Geometry: final body of the model. Coordinates: model frame, mm. A direction names the side the tool comes from. Coordinates: 2 decimals unless noted, no trailing zeros. Loops run counter-clockwise (first coordinate to the right, second up) from the corner with the lowest first, then second, coordinate; pieces in that order, holes last. Notation, with made-up numbers: (56, -6) - (65, -6) arc R27 cw to (65, 16) - close; hole circle Ø7 at (-40, 12.5). An arc over 180 degrees is marked (long way). Answer in a Markdown table with one row per item.
from build123d import *

# Parameters (mm, degrees)
BOSS_EXTRUDE1_DEPTH     = 19.05
SKETCH2_W               = 42.164
SKETCH2_H               = 27.686
BOSS_EXTRUDE2_DEPTH     = 2.54
SKETCH3_W               = 7.0612
SKETCH3_H               = 14.986
BOSS_EXTRUDE3_DEPTH     = 3.175
CUT_EXTRUDE1_DEPTH      = 50.127067096
CUT_EXTRUDE1_DEPTH_BACK = 50.127067096
SKETCH4_R               = 1.75
FILLET2_R               = 1.27
CUT_EXTRUDE2_DEPTH      = 52.65763053
CUT_EXTRUDE2_DEPTH_BACK = 52.65763053
SKETCH5_R               = 4.7625
SKETCH6_W               = 25.4
SKETCH6_H               = 4.7625
BOSS_EXTRUDE4_DEPTH     = 9.525
FILLET3_R               = 3.175
FILLET4_R               = 1.27
FILLET6_R               = 1.27
SKETCH8_R               = 2.3
CUT_EXTRUDE3_DEPTH      = 58.486687197
SKETCH9_W               = 2.54
SKETCH9_H               = 10.16
CUT_EXTRUDE4_DEPTH      = 14.5288
FILLET3_OF_MIRROR2_R    = 3.175
FILLET4_OF_MIRROR2_R    = 1.27
SKETCH11_W              = 43.835439061
SKETCH11_H              = 10.898597795
CUT_EXTRUDE5_DEPTH      = 6.858


with BuildPart() as part:
    # Sketch1 → Boss-Extrude1 (new body)
    with BuildSketch(Plane.XY):
        Polygon((-2.54, 25.146), (39.624, 25.146), (39.624, 22.606), (37.084, 22.606), (0, 22.606), (0, 0), (37.084, 0), (39.624, 0), (39.624, -2.54), (-2.54, -2.54), align=None)
    extrude(amount=BOSS_EXTRUDE1_DEPTH)

    # Sketch2 → Boss-Extrude2 (add)
    with BuildSketch(Plane.XY.offset(19.05)):
        with Locations((18.542, 11.303)):
            Rectangle(SKETCH2_W, SKETCH2_H)
    extrude(amount=BOSS_EXTRUDE2_DEPTH)

    # Sketch3 → Boss-Extrude3 (add)
    with BuildSketch(Plane.ZY.offset(2.54)):
        with Locations((18.0594, 11.303)):
            Rectangle(SKETCH3_W, SKETCH3_H)
    extrude(amount=BOSS_EXTRUDE3_DEPTH)

    # Sketch4 → Cut-Extrude1 (cut, two sides: drawn at the far end of the back side and taken through both)
    with BuildSketch(Plane(origin=(0, 0, 14.5288), x_dir=(-1, 0, 0), z_dir=(0, 0, -1)).offset(-CUT_EXTRUDE1_DEPTH_BACK)):
        with Locations(Location((2.2225, 11.303, 0), (0, 0, 90))):
            Circle(SKETCH4_R)
    extrude(amount=CUT_EXTRUDE1_DEPTH + CUT_EXTRUDE1_DEPTH_BACK, mode=Mode.SUBTRACT)

    # Fillet2
    fillet2_edges = [part.edges().sort_by_distance(p)[0] for p in [
        (-2.54, 18.796, 18.0594),
        (-2.54, 3.81, 18.0594),
        (-5.715, 18.796, 18.0594),
        (-5.715, 3.81, 18.0594),
    ]]
    fillet(fillet2_edges, radius=FILLET2_R)

    # Sketch5 → Cut-Extrude2 (cut, two sides: drawn at the far end of the back side and taken through both)
    with BuildSketch(Plane.XY.offset(21.59).offset(-CUT_EXTRUDE2_DEPTH_BACK)):
        with Locations((10.16, 11.303)):
            Circle(SKETCH5_R)
        with BuildLine():
            Line((25.4, 16.0655), (10.16, 16.0655))
            ThreePointArc((10.16, 16.0655), (13.527596045, 14.670596045), (14.9225, 11.303))
            ThreePointArc((14.9225, 11.303), (13.527596045, 7.935403955), (10.16, 6.5405))
            Line((10.16, 6.5405), (25.4, 6.5405))
            ThreePointArc((25.4, 6.5405), (20.6375, 11.303), (25.4, 16.0655))
        make_face()
        with Locations((25.4, 11.303)):
            Circle(SKETCH5_R)
    extrude(amount=CUT_EXTRUDE2_DEPTH + CUT_EXTRUDE2_DEPTH_BACK, mode=Mode.SUBTRACT)

    # Sketch6 → Boss-Extrude4 (add)
    with BuildSketch(Plane.XY.offset(21.59)):
        with Locations((26.924, 22.76475)):
            Rectangle(SKETCH6_W, SKETCH6_H)
    boss_extrude4 = extrude(amount=BOSS_EXTRUDE4_DEPTH)

    # Fillet3
    fillet3_edges = [part.edges().sort_by_distance(p)[0] for p in [
        (14.224, 22.76475, 21.59),
        (14.224, 22.76475, 31.115),
        (39.624, 22.76475, 31.115),
    ]]
    fillet(fillet3_edges, radius=FILLET3_R)

    # Fillet4
    fillet4_edges = [part.edges().sort_by_distance(p)[0] for p in [
        (25.3365, 20.3835, 21.59),
    ]]
    fillet(fillet4_edges, radius=FILLET4_R)

    # Fillet6
    fillet6_edges = [part.edges().sort_by_distance(p)[0] for p in [
        (0, 0, 9.525),
        (0, 22.606, 9.525),
    ]]
    fillet(fillet6_edges, radius=FILLET6_R)

    # Sketch8 → Cut-Extrude3 (cut, symmetric)
    with BuildSketch(Plane(origin=(0, 25.146, 0), x_dir=(1, 0, 0), z_dir=(0, 1, 0))):
        with Locations(Location((20.574, -26.3525, 0), (0, 0, 270))):
            Circle(SKETCH8_R)
        with Locations(Location((33.274, -26.3525, 0), (0, 0, 270))):
            Circle(SKETCH8_R)
    cut_extrude3 = extrude(amount=CUT_EXTRUDE3_DEPTH, both=True, mode=Mode.SUBTRACT)

    # Sketch9 → Cut-Extrude4 (cut)
    with BuildSketch(Plane(origin=(0, 0, 0), x_dir=(-1, 0, 0), z_dir=(0, 0, -1))):
        with Locations((1.27, 11.303)):
            Rectangle(SKETCH9_W, SKETCH9_H)
    extrude(amount=-CUT_EXTRUDE4_DEPTH, mode=Mode.SUBTRACT)

    # Mirror2: Boss-Extrude4, Cut-Extrude3 across plane
    add(boss_extrude4.mirror(Plane.ZX.offset(11.303)))
    add(cut_extrude3.mirror(Plane.ZX.offset(11.303)), mode=Mode.SUBTRACT)

    # Fillet3 of Mirror2
    fillet3_of_mirror2_edges = [part.edges().sort_by_distance(p)[0] for p in [
        (14.224, -0.15875, 21.59),
        (14.224, -0.15875, 31.115),
        (39.624, -0.15875, 31.115),
    ]]
    fillet(fillet3_of_mirror2_edges, radius=FILLET3_OF_MIRROR2_R)

    # Fillet4 of Mirror2
    fillet4_of_mirror2_edges = [part.edges().sort_by_distance(p)[0] for p in [
        (25.3365, 2.2225, 21.59),
    ]]
    fillet(fillet4_of_mirror2_edges, radius=FILLET4_OF_MIRROR2_R)

    # Sketch11 → Cut-Extrude5 (cut)
    with BuildSketch(Plane(origin=(0, 25.146, 0), x_dir=(1, 0, 0), z_dir=(0, 1, 0))):
        with Locations((19.377719531, -27.039298898)):
            Rectangle(SKETCH11_W, SKETCH11_H)
    extrude(amount=-CUT_EXTRUDE5_DEPTH, mode=Mode.SUBTRACT)


solid = part.part
(1) Pull-direction query (Y, two-part tool) for faces 6 (the face through (-3.93, 10.92, 18.11)), 7 (the face through (38.67, -0.19, 30.21)), 8 (the face through (-5.33, 4.17, 18.11)), 9 (the face through (21, 0, 9)); classes: pulls with the +Y half, pulls with the -Y half, needs draft (parallel to the pull), parting line crosses it, or undercut.
Verdict:
| item | result |
|---|---|
| face 6 | undercut |
| face 7 | needs draft |
| face 8 | pulls with the -Y half |
| face 9 | undercut |
(2) Ray query, probe 1 along Y at (x, z) = (37, 10.5); probe 2 along Y at (x, z) = (-1, 3); probe 3 along X at (y, z) = (20.5, 4). Return the intervals inside material, ascending.
Verdict:
| item | result |
|---|---|
| probe 1 | y = -2.54 to 0, 22.61 to 25.15 |
| probe 2 | y = -2.54 to 6.22, 16.38 to 25.15 |
| probe 3 | x = -2.54 to 0 |
(3) First-contact query: pin 1 Ø1.6 at (y, z) = (0, 27) entering from -X; pin 2 Ø1.5 at (x, z) = (10.5, 22) entering from +Y; pin 3 Ø4.5 at (x, y) = (-2.22, 11.3) entering from -Z; pin 4 Ø7 at (y, z) = (20.5, 9.5) entering from -X. Flat tips, straight axial feed; report the tip coordinate or a pass-through.
Verdict:
| item | result |
|---|---|
| pin 1 | stops at x = 14.22 |
| pin 2 | stops at y = 25.15 |
| pin 3 | stops at z = 14.53 |
| pin 4 | stops at x = -2.54 |
(4) Access query for faces 1 (the face through (-2.54, 2, 8)), 2 (the face through (14.224, 0, 26)), 3 (the face through (-1, 16.383, 7)), 4 (the face through (18, 6.54, 20)), 5 (the face through (0, 11, 16)). Directions: +Z, -Z, +X, -X, +Y, -Y. A direction counts if a zero-diameter tool reaches every point of the face in a straight line with its end or side. Return the directions, or none.
Verdict:
| item | result |
|---|---|
| face 1 | -Z, -X, -Y |
| face 2 | +Z, -X, +Y, -Y |
| face 3 | -Z, +X, -X |
| face 4 | +Z, -Z |
| face 5 | -Z, +X |
(5) Cut plane A-A on z = 12.5. Output: boundary loops of the cut face in (x, y), then the cut area to 3 significant figures.
Verdict:
| item | result |
|---|---|
| outline | (-2.54, -2.54) - (39.62, -2.54) - (39.62, 0) - (1.27, 0) arc R1.27 cw to (0, 1.27) - (0, 6.22) - (-2.54, 6.22) - close; (-2.54, 16.38) - (0, 16.38) - (0, 21.34) arc R1.27 cw to (1.27, 22.61) - (39.62, 22.61) - (39.62, 25.15) - (-2.54, 25.15) - close |
| area | 246 mm² |
(6) Cut plane D-D on x = 6.5. Output: boundary loops of the cut face in (y, z).
Verdict:
| item | result |
|---|---|
| outline | (-2.54, 0) - (0, 0) - (0, 19.05) - (8.26, 19.05) - (8.26, 21.59) - (-2.54, 21.59) - close; (14.35, 19.05) - (22.61, 19.05) - (22.61, 0) - (25.15, 0) - (25.15, 21.59) - (14.35, 21.59) - close |
